```python
from build123d import *

# Parameters (mm, degrees)
F1_DEPTH = 14.37
F0_R     = 2
F2_DEPTH = 7.185
F3_R     = 2.05
F4_DEPTH = 7.185


with BuildPart() as f1:
    # F0 (on Front) → F1 (new body)
    with BuildSketch(Plane.XZ):
        with BuildLine():
            ThreePointArc((7.1321428571, 0.3034947896), (7.7481620558, 0.0769305381), (8.4, 0))
            Line((8.4, 0), (16.6, 0))
            ThreePointArc((16.6, 0), (17.2518379442, 0.0769305381), (17.8678571429, 0.3034947896))
            ThreePointArc((17.8678571429, 0.3034947896), (18.9864199128, 1.3354181484), (19.4, 2.8))
            ThreePointArc((19.4, 2.8), (20.2201010127, 4.7798989873), (22.2, 5.6))
            Line((22.2, 5.6), (22.2, 6.7))
            ThreePointArc((22.2, 6.7), (21.8778174593, 5.9221825407), (21.1, 5.6))
            Line((21.1, 5.6), (18.0575369646, 5.6))
            Line((18.0575369646, 5.6), (6.9424630354, 5.6))
            Line((6.9424630354, 5.6), (3.9, 5.6))
            Line((3.9, 5.6), (2.8, 5.6))
            ThreePointArc((2.8, 5.6), (4.7798989873, 4.7798989873), (5.6, 2.8))
            ThreePointArc((5.6, 2.8), (6.0135800872, 1.3354181484), (7.1321428571, 0.3034947896))
        make_face()
        with BuildLine():
            ThreePointArc((20.2574998019, 7.4072435339), (19.0261653027, 6.6635182559), (18.0575369646, 5.6))
            Line((18.0575369646, 5.6), (21.1, 5.6))
            ThreePointArc((21.1, 5.6), (20.103012566, 6.2352247249), (20.2574998019, 7.4072435339))
        make_face()
        with BuildLine():
            ThreePointArc((20.2574998019, 7.4072435339), (20.103012566, 6.2352247249), (21.1, 5.6))
            ThreePointArc((21.1, 5.6), (21.8778174593, 5.9221825407), (22.2, 6.7))
            ThreePointArc((22.2, 6.7), (21.9926506427, 7.3427867688), (21.4487730361, 7.7432436768))
            ThreePointArc((21.4487730361, 7.7432436768), (20.8426991749, 7.6122483799), (20.2574998019, 7.4072435339))
        make_face()
        with BuildLine():
            ThreePointArc((4.7425001981, 7.4072435339), (4.896987434, 6.2352247249), (3.9, 5.6))
            Line((3.9, 5.6), (6.9424630354, 5.6))
            ThreePointArc((6.9424630354, 5.6), (5.9738346973, 6.6635182559), (4.7425001981, 7.4072435339))
        make_face()
        with BuildLine():
            ThreePointArc((2.8, 6.7), (3.1221825407, 5.9221825407), (3.9, 5.6))
            ThreePointArc((3.9, 5.6), (4.896987434, 6.2352247249), (4.7425001981, 7.4072435339))
            ThreePointArc((4.7425001981, 7.4072435339), (4.1573008251, 7.6122483799), (3.5512269639, 7.7432436768))
            ThreePointArc((3.5512269639, 7.7432436768), (3.0073493573, 7.3427867688), (2.8, 6.7))
        make_face()
        with BuildLine():
            Line((2.8, 6.7), (2.8, 5.6))
            Line((2.8, 5.6), (3.9, 5.6))
            ThreePointArc((3.9, 5.6), (3.1221825407, 5.9221825407), (2.8, 6.7))
        make_face()
    extrude(amount=F1_DEPTH)



with BuildPart() as f1b:
    # F0 (on Front) → F1, piece 2 (new body)
    with BuildSketch(Plane.XZ):
        with Locations((22.2, 2.8)):
            Circle(F0_R)
    extrude(amount=F1_DEPTH)


with BuildPart() as f1_1:
    add(f1.part)

    add(f1b.part)  # F2 merges F1b
    # F0 (on Front) → F2 (join)
    with BuildSketch(Plane.XZ):
        with BuildLine():
            ThreePointArc((17.8678571429, 0.3034947896), (17.2518379442, 0.0769305381), (16.6, 0))
            Line((16.6, 0), (22.2, 0))
            ThreePointArc((22.2, 0), (20.2201010127, 0.8201010127), (19.4, 2.8))
            ThreePointArc((19.4, 2.8), (18.9864199128, 1.3354181484), (17.8678571429, 0.3034947896))
        make_face()
        with BuildLine():
            ThreePointArc((19.4, 2.8), (20.2201010127, 0.8201010127), (22.2, 0))
            ThreePointArc((22.2, 0), (24.1798989873, 0.8201010127), (25, 2.8))
            ThreePointArc((25, 2.8), (24.1798989873, 4.7798989873), (22.2, 5.6))
            ThreePointArc((22.2, 5.6), (20.2201010127, 4.7798989873), (19.4, 2.8))
        make_face()
        with Locations((22.2, 2.8)):
            Circle(F0_R, mode=Mode.SUBTRACT)
    extrude(amount=F2_DEPTH)

    # F3 (on face) → F4 (join)
    with BuildSketch(Plane.XZ.offset(14.37)):
        with BuildLine():
            ThreePointArc((2.8, 0), (4.7798989873, 0.8201010127), (5.6, 2.8))
            ThreePointArc((5.6, 2.8), (4.7798989873, 4.7798989873), (2.8, 5.6))
            ThreePointArc((2.8, 5.6), (0, 2.8), (2.8, 0))
        make_face()
        with Locations((2.8, 2.8)):
            Circle(F3_R, mode=Mode.SUBTRACT)
        with BuildLine():
            ThreePointArc((8.4, 0), (6.4201010127, 0.8201010127), (5.6, 2.8))
            ThreePointArc((5.6, 2.8), (4.7798989873, 0.8201010127), (2.8, 0))
            Line((2.8, 0), (8.4, 0))
        make_face()
    extrude(amount=-F4_DEPTH)


solid = f1_1.part
```
Part model, mm, in its own coordinate system. A direction names the side the tool comes from. Round coordinates to 2 decimals unless told otherwise and drop trailing zeros. Loops run counter-clockwise (first coordinate to the right, second up) from the corner with the lowest first, then second, coordinate; pieces in that order, holes last. Notation, with made-up numbers: (87, 55.25) -> (133, 55.25) arc R23 ccw to (133, 92.25) -> close; hole circle Ø11 at (62.5, 31). An arc over 180 degrees is marked (long way). Use CSV: the item, a comma, the result in double quotes. Start each with the question number.
1) Cut at B-B, the plane z = 3.25. Write the cut outline in (x, y) (3 decimals).
2) Wall check: L1, parallel to X at y = -7.75, z = 2.5; L2, parallel to X at y = -8.5, z = 7; L3, parallel to X at y = -8.75, z = 5.75. Give the ranges that are in metal, low to high. Write a range as [from, to].
3) Cut at A-A, the plane y = -11.5. Write the cut outline in (x, z), plus the area to 3 significant figures.
4) Pull direction X, two halves, no side cores. Call faces 1 (the cylindrical face through (0.75, -10.83, 2.89)), 2 (the flat face through (14, 0, 3)), 3 (the flat face through (22.2, -7, 6)): +X half, -X half, draft (parallel to the pull), parting line (faces both ways), or undercut.
5) Which spindle directions (+Z, -Z, +X, -X, +Y, -Y) get a long thin tool onto all of the face, cutting with end or side? Do faces 4 (the flat face through (13, -7, 5.6)), 5 (the flat face through (22, -14.37, 3)), 6 (the flat face through (5, -7.185, 2)), 7 (the cylindrical face through (24.108, -10.727, 3.401)), 8 (the flat face through (2.8, -7, 6)). Say none if no direction does.
6) Drop flat-ended pins along their axis: P1, Ø3, axis at x = 11.5, y = -6.5, coming from the +Z side; P2, Ø2.5, axis at x = 2.8, z = 2.8, coming from the +Y side; P3, Ø1.5, axis at y = -5, z = 5, coming from the -X side; P4, Ø1.2, axis at y = -5.5, z = 6.5, coming from the +X side. Give the stop position or say it passes through.
7) Cut at C-C, the plane y = -3.5. Write the cut outline in (x, z).
8) Cut at D-D, the plane x = 22.75. Write the cut outline in (y, z) (3 decimals).
Determined:
1,outline,"(0.036, -14.37) -> (0.8, -14.37) -> (0.8, -7.185) -> (0.036, -7.185) -> close; (4.8, -14.37) -> (19.436, -14.37) -> (19.436, -7.185) -> (20.251, -7.185) -> (20.251, -14.37) -> (24.149, -14.37) -> (24.149, -7.185) -> (24.964, -7.185) -> (24.964, 0) -> (5.564, 0) -> (5.564, -7.185) -> (4.8, -7.185) -> close"
2,L1,"x = [0.02, 0.77], [4.83, 19.38], [20.22, 24.18]"
2,L2,"x = [2.84, 5.51], [19.49, 22.16]"
2,L3,"x = [2.8, 6.84], [18.16, 22.2]"
3,outline,"(2.8, 0) -> (16.6, 0) arc R2.8 ccw to (19.4, 2.8) arc R2.8 cw to (22.2, 5.6) -> (22.2, 6.7) arc R1.1 ccw to (21.45, 7.74) arc R5 ccw to (18.06, 5.6) -> (6.94, 5.6) arc R5 ccw to (3.55, 7.74) arc R1.1 ccw to (2.8, 6.7) -> (2.8, 5.6) arc R2.8 ccw to start; circle Ø4 at (22.2, 2.8); hole circle Ø4.1 at (2.8, 2.8)"
3,area,"117 mm2"
4,face 1,"undercut"
4,face 2,"draft"
4,face 3,"+X half"
5,face 4,"+Z, +Y, -Y"
5,face 5,"+Z, -Z, +X, -X, -Y"
5,face 6,"-Z, -X, +Y"
5,face 7,"-Y"
5,face 8,"+Z, -X, +Y, -Y"
6,P1,"stops at z = 5.6"
6,P2,"passes through"
6,P3,"stops at x = 2.8"
6,P4,"stops at x = 22.2"
7,outline,"(2.8, 5.6) arc R2.8 cw to (5.6, 2.8) arc R2.8 ccw to (8.4, 0) -> (22.2, 0) arc R2.8 ccw to (22.2, 5.6) -> (22.2, 6.7) arc R1.1 ccw to (21.45, 7.74) arc R5 ccw to (18.06, 5.6) -> (6.94, 5.6) arc R5 ccw to (3.55, 7.74) arc R1.1 ccw to (2.8, 6.7) -> close"
8,outline,"(-14.37, 0.877) -> (-7.185, 0.877) -> (-7.185, 0.055) -> (0, 0.055) -> (0, 5.545) -> (-7.185, 5.545) -> (-7.185, 4.723) -> (-14.37, 4.723) -> close"
